Build history of the part. All positions in model axes, mm. Face numbers are marked on the shaded views. A direction names the side the tool comes from. Give positions to 0.01 mm unless a question says otherwise; leave off trailing zeros. Order: outer loops, then holes, each group sorted by start corner. A loop starts at its lowest first (then second) coordinate and runs counter-clockwise, first axis right, second up. Notation, with made-up numbers: M 83.25,24 L 115.25,24 A12 ccw 115.25,32 Z; hole C -33.75,23.25 d7. An arc over 180 degrees is marked long. One line per item, written item: value. Start each with the question number.
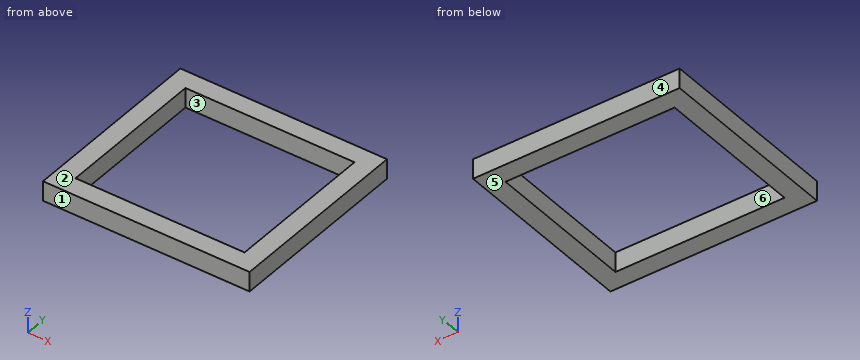
Autodesk Fusion 360 part; units mm, degrees
sketch "Sketch1" plane through (0, 0, 0) normal (0, 0, 1) x (1, 0, 0)
  line L0 (0, 0) -> (41.91, 0)
  line L1 (41.91, 0) -> (41.91, 38.1)
  line L2 (41.91, 38.1) -> (0, 38.1)
  line L3 (0, 38.1) -> (0, 0)
  line L4 (0, 38.1) -> (3.81, 38.1)
  line L5 (3.81, 34.29) -> (3.81, 3.81)
  line L6 (0, 0) -> (0, 3.81)
  line L7 (3.81, 3.81) -> (38.1, 3.81)
  line L8 (0, 38.1) -> (0, 34.29)
  line L9 (3.81, 34.29) -> (38.1, 34.29)
  line L10 (41.91, 38.1) -> (38.1, 38.1)
  line L11 (38.1, 34.29) -> (38.1, 3.81)
  dimension "d1" = 41.91
  dimension "d2" = 38.1
  dimension "d3" = 3.81
  dimension "d4" = 3.81
  dimension "d5" = 3.81
  dimension "d6" = 3.81
sketch "Sketch2" plane through (0, 0, 0) normal (0, 0, 1) x (1, 0, 0)
extrude "Extrude1" add sketch "Sketch1" along normal blind 4
1) Tool access for the marked faces 5 and 6: list every direction of +Z, -Z, +X, -X, +Y, -Y with a clear straight run to the whole face (end or side of a thin tool).
2) Slice it at B-B (y = 30.5). List the corners of the cut face in (x, z).
3) Pull direction Y, two halves, no side cores. Call the marked faces 1, 2, 3 and 4: pulls with the +Y half, pulls with the -Y half, needs draft (parallel to the pull), parting line crosses it, or undercut.
4) Slice it at A-A (x = 15). List the corners of the cut face in (y, z).
5) Drop flat-ended pins along their axis: P1, Ø1, axis at x = 36.5, z = 1, coming from the -Y side; P2, Ø1, axis at x = 4.5, y = 27.5, coming from the -Z side. Give the stop position or say it passes through.
6) Drill centre lines: line 1 (X direction, y = 8, z = 0.95); line 2 (Y direction, x = 19, z = 3.2). Where is each one in solid material? Low to high.
7) Slice it at C-C (z = 1.9). List the corners of the cut face in (x, y).
Results list:
1. face 5: -Z, +X, -X, +Y, -Y
1. face 6: +Z, -Z
2. outline: M 0,0 L 3.81,0 L 3.81,4 L 0,4 Z; M 38.1,0 L 41.91,0 L 41.91,4 L 38.1,4 Z
3. face 1: pulls with the -Y half
3. face 2: needs draft
3. face 3: undercut
3. face 4: pulls with the +Y half
4. outline: M 0,0 L 3.81,0 L 3.81,4 L 0,4 Z; M 34.29,0 L 38.1,0 L 38.1,4 L 34.29,4 Z
5. P1: stops at y = 0
5. P2: passes through
6. line 1: x = 0 to 3.81, 38.1 to 41.91
6. line 2: y = 0 to 3.81, 34.29 to 38.1
7. outline: M 0,0 L 41.91,0 L 41.91,38.1 L 0,38.1 Z; hole M 3.81,3.81 L 38.1,3.81 L 38.1,34.29 L 3.81,34.29 Z
